Solid Edge part; units mm, degrees
sketch "Sketch1" plane through (0, 0, 0) normal (0, 0, 1) x (1, 0, 0)
  line L0 (-10, -10) -> (10, -10)
  line L1 (10, -10) -> (10, 10)
  line L2 (10, 10) -> (-10, 10)
  line L3 (-10, 10) -> (-10, -10)
  circle A0 centre (0, 0) radius 5
  dimension "D1" = 10
extrude "Protrusion1" add sketch "Sketch1" along normal blind 1
pattern_linear "Pattern1" count 15 spacing 20 along (1, 0, 0) count 4 spacing 20 along (0, -1, 0) of "Protrusion1"
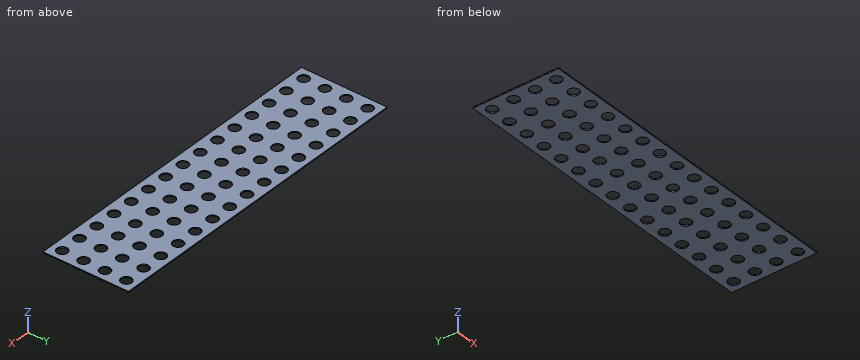
The listing builds one solid part. Answer for the finished solid, in the listing's coordinates (mm). Round coordinates to 2 decimals unless told otherwise and drop trailing zeros. Write each loop counter-clockwise with the first axis right and the second up, starting at its lowest first coordinate (ties: lowest second). Pieces come first, ordered by that corner, then holes. Notation, with made-up numbers: (23.5, 16.5) - (59.5, 16.5) arc R9 ccw to (59.5, 28.5) - close; hole circle Ø5 at (79.25, 44). An arc over 180 degrees is marked (long way). Use a Markdown table: item, result. Add a question column.
1. The part is cut by section D-D (x = 41.5). Write down the section's boundary in (y, z).
2. A flat-ended cylindrical pin translates along its axis: P1, Ø9, axis at x = 240, y = -40, coming from the +Z side. Find the tip coordinate at first contact, or state that the pin passes through.
3. Consider line 1 (Y direction, x = 0, z = 0.8); line 2 (Y direction, x = 23, z = 0.25). Determine where each line is inside the solid, lowest interval first.
4. The part is cut by section A-A (x = 0). Write down the section's boundary in (y, z).
5. The part is cut by section B-B (y = -40). Give the number of separate pieces and of enclosed holes in the cut face, and give its area (3 significant figures).
Reported:
| question | item | result |
|---|---|---|
| 1 | outline | (-70, 0) - (-64.77, 0) - (-64.77, 1) - (-70, 1) - close; (-55.23, 0) - (-44.77, 0) - (-44.77, 1) - (-55.23, 1) - close; (-35.23, 0) - (-24.77, 0) - (-24.77, 1) - (-35.23, 1) - close; (-15.23, 0) - (-4.77, 0) - (-4.77, 1) - (-15.23, 1) - close; (4.77, 0) - (10, 0) - (10, 1) - (4.77, 1) - close |
| 2 | P1 | through |
| 3 | line 1 | -70 to -65, -55 to -45, -35 to -25, -15 to -5, 5 to 10 |
| 3 | line 2 | -70 to -64, -56 to -44, -36 to -24, -16 to -4, 4 to 10 |
| 4 | outline | (-70, 0) - (-65, 0) - (-65, 1) - (-70, 1) - close; (-55, 0) - (-45, 0) - (-45, 1) - (-55, 1) - close; (-35, 0) - (-25, 0) - (-25, 1) - (-35, 1) - close; (-15, 0) - (-5, 0) - (-5, 1) - (-15, 1) - close; (5, 0) - (10, 0) - (10, 1) - (5, 1) - close |
| 5 | separate pieces | 16 |
| 5 | enclosed holes | 0 |
| 5 | area | 150 mm^2 |
